Autodesk Inventor part; units mm, degrees
ref_plane "YZ Plane" through (0, 0, 0) normal (1, 0, 0) x (0, 1, 0)
ref_plane "XZ Plane" through (0, 0, 0) normal (0, 1, 0) x (-1, 0, 0)
ref_plane "XY Plane" through (0, 0, 0) normal (0, 0, 1) x (1, 0, 0)
sketch "Sketch1" plane through (0, 0, 0) normal (0, 0, 1) x (1, 0, 0)
  line L0 (0, 0) -> (65, 0)
  line L1 (65, 0) -> (65, 5.8)
  line L2 (65, 5.8) -> (0, 5.8)
  line L3 (0, 5.8) -> (0, 0)
  line L4 (0, 0) -> (0, 2.9)
  line L5 (0, 2.9) -> (5, 2.9)
  line L6 (5, 2.9) -> (13.2178, 2.9)
  circle A0 centre (5, 2.9) radius 1
  circle A1 centre (13.2178, 2.9) radius 1
  line L7 (13.2178, 2.9) -> (19.2178, 2.9)
  line L8 (19.2178, 2.9) -> (60, 2.9)
  circle A2 centre (19.2178, 2.9) radius 1
  circle A3 centre (60, 2.9) radius 1
  line L9 (19.2178, 3.9) -> (60, 3.9)
  line L10 (60, 1.9) -> (19.2178, 1.9)
  point P0 (65, 2.9)
  dimension "d0" = 65
  dimension "d1" = 5.8
  dimension "d2" = 2.9
  dimension "d3" = 5
  dimension "d4" = 8.2178
  dimension "d5" = 2
  dimension "d6" = 2
  dimension "d7" = 6
  dimension "d8" = 5
  dimension "d9" = 2
  dimension "d10" = 2
extrude "Extrusion1" add sketch "Sketch1" along normal blind 5
fillet "Fillet1" radius 2 4 edges at (0, 5.8, 2.5) (65, 5.8, 2.5) (65, 0, 2.5) (0, 0, 2.5)
sketch "Sketch2" plane through (0, 0, 5) normal (0, 0, 1) x (1, 0, 0)
  arc A0 (0, 2) -> (2, 0) centre (2, 2) ccw
  line L0 (2, 0) -> (63, 0)
  arc A1 (63, 0) -> (65, 2) centre (63, 2) ccw
  line L1 (65, 2) -> (65, 3.8)
  arc A2 (65, 3.8) -> (63, 5.8) centre (63, 3.8) ccw
  line L2 (63, 5.8) -> (2, 5.8)
  arc A3 (2, 5.8) -> (0, 3.8) centre (2, 3.8) ccw
  line L3 (0, 3.8) -> (0, 2)
  arc A4 (19.2178, 3.9) -> (19.2178, 1.9) centre (19.2178, 2.9) ccw
  line L4 (19.2178, 3.9) -> (60, 3.9)
  arc A5 (60, 1.9) -> (60, 3.9) centre (60, 2.9) ccw
  line L5 (60, 1.9) -> (19.2178, 1.9)
  circle A6 centre (13.2178, 2.9) radius 1
  circle A7 centre (5, 2.9) radius 1
  circle A8 centre (5, 2.9) radius 2
  circle A9 centre (13.2178, 2.9) radius 2
  point P0 (0, 0)
  dimension "d14" = 4
  dimension "d15" = 4
extrude "Extrusion2" cut sketch "Sketch2" against normal blind 3 contours A7 | A8 | A9
equation "\"d2\" = 0.5 * d1"
equation "\"d6\" = d5"
equation "\"d7\" = d8 + 0.5 * d5"
equation "\"d9\" = d5"
equation "\"d10\" = d5"
equation "\"d15\" = d14"
properties part number "Locking Lever"
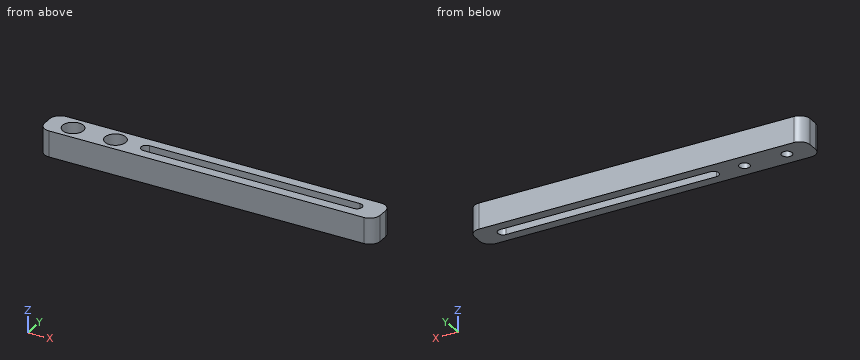
Could you check a few things on this model? Use its own coordinates, in mm. Coordinates: 2 decimals unless noted, no trailing zeros. Write each loop counter-clockwise with the first axis right and the second up, starting at its lowest first coordinate (ties: lowest second). Pieces come first, ordered by that corner, then holes. Notation, with made-up numbers: (35, 46) -> (78, 46) arc R26 ccw to (78, 61) -> close; hole circle Ø6 at (28.5, 29.5). An arc over 180 degrees is marked (long way). Return JSON: item names as keys, results as strings.
(1) I need wall thicknesses on L1, parallel to Y at x = 21, z = 2.8; L2, parallel to X at y = 2.85, z = 0.55; L3, parallel to Y at x = 5, z = 4.15. Which ranges of each line are inside material? Lowest first, please.
Numbers:
{"L1": "y = 0 to 1.9, 3.9 to 5.8", "L2": "x = 0 to 4, 6 to 12.22, 14.22 to 18.22, 61 to 65", "L3": "y = 0 to 0.9, 4.9 to 5.8"}
(2) I'm going to push a flat-ended pin straight in: pin 1 (2 mm diameter, centred on x = 14, y = 2.5, fed in from +Z). Where does the tip first touch, or does it pass through?
Numbers:
{"pin 1": "stops at z = 2"}
(3) Imagine slicing it at A-A, the plane y = 2.9. Please give me the cut outline in (x, z), then the cut area to 3 significant figures.
Numbers:
{"outline": "(0, 0) -> (4, 0) -> (4, 2) -> (3, 2) -> (3, 5) -> (0, 5) -> close; (6, 0) -> (12.22, 0) -> (12.22, 2) -> (11.22, 2) -> (11.22, 5) -> (7, 5) -> (7, 2) -> (6, 2) -> close; (14.22, 0) -> (18.22, 0) -> (18.22, 5) -> (15.22, 5) -> (15.22, 2) -> (14.22, 2) -> close; (61, 0) -> (65, 0) -> (65, 5) -> (61, 5) -> close", "area": "79.1 mm2"}
(4) Imagine slicing it at B-B, the plane x = 44. Please give me the cut outline in (y, z).
Numbers:
{"outline": "(0, 0) -> (1.9, 0) -> (1.9, 5) -> (0, 5) -> close; (3.9, 0) -> (5.8, 0) -> (5.8, 5) -> (3.9, 5) -> close"}
(5) Imagine slicing it at D-D, the plane x = 5. Please give me the cut outline in (y, z).
Numbers:
{"outline": "(0, 0) -> (1.9, 0) -> (1.9, 2) -> (0.9, 2) -> (0.9, 5) -> (0, 5) -> close; (3.9, 0) -> (5.8, 0) -> (5.8, 5) -> (4.9, 5) -> (4.9, 2) -> (3.9, 2) -> close"}
(6) Imagine slicing it at C-C, the plane z = 4.05. Please give me the cut outline in (x, y), then the cut area to 3 significant figures.
Numbers:
{"outline": "(0, 2) arc R2 ccw to (2, 0) -> (63, 0) arc R2 ccw to (65, 2) -> (65, 3.8) arc R2 ccw to (63, 5.8) -> (2, 5.8) arc R2 ccw to (0, 3.8) -> close; hole circle Ø4 at (5, 2.9); hole circle Ø4 at (13.22, 2.9); hole (19.22, 1.9) -> (60, 1.9) arc R1 ccw to (60, 3.9) -> (19.22, 3.9) arc R1 ccw to start", "area": "264 mm2"}
